Verification items for this drawing (mm, ordinates from the low corner). A direction names the side the tool comes from. Coordinates: 2 decimals unless noted, no trailing zeros. Loops run counter-clockwise (first coordinate to the right, second up) from the corner with the lowest first, then second, coordinate; pieces in that order, holes last. Notation, with made-up numbers: M 39,24.25 L 96,24.25 A23 cw 96,50.25 Z; hole C 70.25,74 d3. An arc over 180 degrees is marked long. One line per question, with ' | ' between items. Start each with the question number.
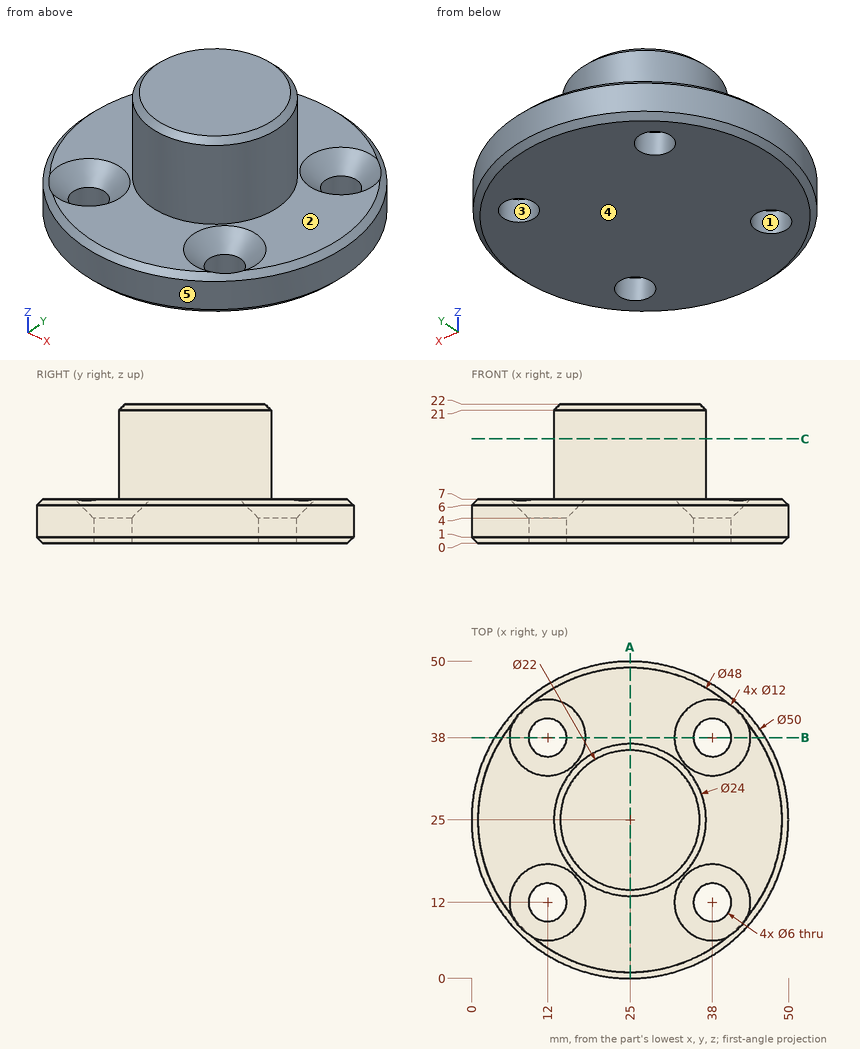
1. Sectioned sample at A-A (x = 25). Record the cut outline in (y, z), and give its area (3 significant figures).
2. Depth check by flat-ended pin: pin 1 Ø8 at (x, y) = (12, 38) entering from -Z; pin 2 Ø5 at (x, y) = (12, 12) entering from +Z; pin 3 Ø4 at (x, z) = (39, 4) entering from -Y; pin 4 Ø10 at (y, z) = (40.5, 16.5) entering from -X. Enter the tip coordinate at first touch or a pass-through.
3. Sectioned sample at B-B (y = 38). State how many separate pieces and enclosed holes the cut face has, and give its area (3 significant figures).
4. Draft check along Y on the marked faces 3, 4 and 5. Enter one of: +Y half, -Y half, draft (parallel to the pull), parting line (faces both ways), or undercut.
5. Thickness scan on line 1 (Y direction, x = 12, z = 2.25); line 2 (Z direction, x = 28, y = 12.5); line 3 (Y direction, x = 38, z = 0.95). Record the ranges inside material, lowest first.
6. Tool access check on the marked faces 1 and 2. Record the directions out of +Z, -Z, +X, -X, +Y, -Y that give a thin tool (end or side, any length) a straight path to the whole face; none if there is none.
7. Sectioned sample at C-C (z = 16.5). Record the cut outline in (x, y).
Result:
1) outline: M 0,1 L 1,0 L 49,0 L 50,1 L 50,6 L 49,7 L 37,7 L 37,21 L 36,22 L 14,22 L 13,21 L 13,7 L 1,7 L 0,6 Z | area: 707 mm2
2) pin 1: stops at z = 0 | pin 2: passes through | pin 3: stops at y = 3.07 | pin 4: stops at x = 19.19
3) separate pieces: 3 | enclosed holes: 0 | area: 195 mm2
4) face 3: undercut | face 4: draft | face 5: parting line
5) line 1: y = 3.65 to 9, 15 to 35, 41 to 46.35 | line 2: z = 0 to 7 | line 3: y = 3.7 to 9, 15 to 35, 41 to 46.3
6) face 1: +Z, -Z | face 2: +Z
7) outline: C 25,25 d24
